Autodesk Inventor part; units mm, degrees
ref_plane "YZ Plane" through (0, 0, 0) normal (1, 0, 0) x (0, 1, 0)
ref_plane "XZ Plane" through (0, 0, 0) normal (0, 1, 0) x (-1, 0, 0)
ref_plane "XY Plane" through (0, 0, 0) normal (0, 0, 1) x (1, 0, 0)
sketch "スケッチ1" plane through (0, 0, 0) normal (0, 0, 1) x (1, 0, 0)
  arc A0 (0.7632, 11.9121) -> (-1.0179, 11.893) centre (0, 0) ccw construction
  arc A1 (0.4062, 11.3607) -> (-0.4062, 11.3607) centre (0, 0) ccw
  arc A2 (9.3048, 1.5803) -> (-9.0567, 2.6555) centre (0, 0) ccw construction
  arc A3 (0.8923, 10.7753) -> (1.9623, 9.2318) centre (2.2471, 10.5718) ccw
  line L0 (1.9623, 9.2318) -> (0, 0)
  arc A4 (-1.9623, 9.2318) -> (-0.8923, 10.7753) centre (-2.2471, 10.5718) ccw
  line L1 (-1.9623, 9.2318) -> (0, 0)
  arc A5 (-0.4062, 11.3607) -> (-0.8923, 10.7753) centre (-0.388, 10.8511) ccw
  arc A6 (0.8923, 10.7753) -> (0.4062, 11.3607) centre (0.388, 10.8511) ccw
  line L2 (0, 0) -> (0, 2.9942) construction
  dimension "d0" = 11.9365
  dimension "d1" = 11.368
  dimension "d2" = 1.93
  dimension "d3" = 0.51
  dimension "d4" = 1.37
  dimension "d5" = 1.37
  dimension "d6" = 24
  dimension "d7" = 12
extrude "押し出し1" add sketch "スケッチ1" along normal blind 11
pattern_circular "円形状パターン1" count 15 over 360 about axis through (0, 0, 0) along (0, 0, 1) of "押し出し1"
sketch "スケッチ3" plane through (0, 0, 0) normal (0, 0, -1) x (-1, 0, 0)
  circle A0 centre (0, 0) radius 13
  dimension "d16" = 26
extrude "押し出し3" add sketch "スケッチ3" along normal blind 2
sketch "スケッチ4" plane through (0, 0, -2) normal (0, 0, -1) x (-1, 0, 0)
  circle A0 centre (0, 0) radius 4.25
  circle A1 centre (-7, 0) radius 1.6
  circle A2 centre (7, 0) radius 1.6
  circle A3 centre (0, 7) radius 1.6
  circle A4 centre (0, -7) radius 1.6
  dimension "d19" = 8.5
  dimension "d20" = 3.2
  dimension "d21" = 3.2
  dimension "d22" = 3.2
  dimension "d23" = 14
  dimension "d24" = 7
  dimension "d25" = 7
  dimension "d26" = 3.2
  dimension "d27" = 7
extrude "押し出し4" cut sketch "スケッチ4" against normal through all
fillet "フィレット1" radius 1 3 edges at (13, 0, 0) (13, 0, -2) (4.25, 0, -2)
properties part number "プーリ_歯数15_3Dプリンタ"
Geometry check sheet. Reference: the model listing, model coordinates, mm. A direction names the side the tool comes from. Give positions to 0.01 mm unless a question says otherwise; leave off trailing zeros. Write item = value, one per line.
(1) Tool access check on faces 4 (the face through (2.97, 9.41, 5.42)), 5 (the face through (-1, 10, 5)), 6 (the face through (8.023, 5.704, 5.423)). Record the directions out of +Z, -Z, +X, -X, +Y, -Y that give a thin tool (end or side, any length) a straight path to the whole face; none if there is none.
Answer below:
face_4 = +Z, +Y
face_5 = +Z
face_6 = +Z, +X
(2) Gauge pin test, flat ends, axial feed: pin 1 Ø5 at (x, z) = (-6, 7) entering from +Y; pin 2 Ø1 at (y, z) = (-8, 5) entering from +X; pin 3 Ø1.9 at (x, y) = (-7, 0) entering from +Z; pin 4 Ø3.5 at (x, y) = (0, 7) entering from -Z. Record the tip position at first contact, or that the pin passes through.
Answer below:
pin_1 = 10.58
pin_2 = 7.2
pin_3 = through
pin_4 = -2
(3) Release check for a two-part mould opening along Y. For faces 1 (the face through (-2.285, 3.584, 4.916)), 2 (the face through (-6.512, 7.383, 5.423)), 3 (the face through (-4.9, -8.6, 5.4)) record: released by +Y, released by -Y, zero draft, split by the parting line, or undercut.
Answer below:
face_1 = undercut
face_2 = released by +Y
face_3 = released by -Y
(4) Material ranges on line 1 (Y direction, x = 0, z = 6.25); line 2 (Y direction, x = -7, z = 4); line 3 (X direction, y = -0.5, z = 0.5), recorded low to high. Write a range as [from, to].
Answer below:
line_1 = [-9.44, -8.6], [-5.4, -4.25], [4.25, 5.4], [8.6, 11.37]
line_2 = [-8.96, -8.13], [-6.33, -1.6], [1.6, 7.54]
line_3 = [-11.28, -8.52], [-5.48, -4.22], [4.22, 5.48], [8.52, 11.28]
(5) Sectioned sample at A-A, the plane z = 3.25. State how many separate pieces and enclosed holes the cut face has, plus the area to 3 significant figures.
Answer below:
separate_pieces = 1
enclosed_holes = 5
area = 249 mm2
